```python
from build123d import *

# Parameters (mm, degrees)
F2_T     = -30.48
F3_DEPTH = 50.8
F4_R     = 12.7


with BuildPart() as f1:
    # F0 (on Front) → F1 (revolve)
    with BuildSketch(Plane.XZ):
        Polygon((-152.4, 0), (0, 0), (0, 152.4), (-208.28, 152.4), align=None)
    revolve(axis=Axis((0, 0, 76.2), (0, 0, -1)))

    # F2
    f2_openings = [f1.faces().sort_by_distance(p)[0] for p in [
        (0, 0, 152.4),
    ]]
    offset(amount=F2_T, openings=f2_openings)

    # F3 (add): a face of the model
    f3_faces = [f1.faces().sort_by_distance(p)[0] for p in [
        (202.3889519846, 0, 152.4),
    ]]
    extrude(f3_faces, amount=F3_DEPTH)

    # F4
    f4_edges = [f1.edges().sort_by_distance(p)[0] for p in [
        (208.28, 0, 203.2),
        (175.81566, 0, 203.2),
        (175.81566, 0, 152.4),
        (208.28, 0, 152.4),
        (152.4, 0, 0),
    ]]
    fillet(f4_edges, radius=F4_R)


solid = f1.part
```
Check sheet for the modelled part. Datum: model origin and axes. Units: mm. A direction names the side the tool comes from. Round coordinates to 2 decimals unless told otherwise and drop trailing zeros. Order: outer loops, then holes, each group sorted by start corner. A loop starts at its lowest first (then second) coordinate and runs counter-clockwise, first axis right, second up. Notation, with made-up numbers: (50, 8) -> (54, 8) arc R33 cw to (54, 43) -> close; hole circle Ø7 at (78, 75). An arc over 180 degrees is marked (long way). Use CSV: the item, a comma, the result in double quotes.
(1) Cross-section at B-B (z = 113). Record the boundary of the cut face in (x, y), and give its area (3 significant figures).
Worked out:
outline,"circle Ø387.67 at (0, 0); hole circle Ø322.74 at (0, 0)"
area,"36,200 mm²"
(2) Cross-section at A-A (z = 169). Record the boundary of the cut face in (x, y).
Worked out:
outline,"circle Ø416.56 at (0, 0); hole circle Ø351.63 at (0, 0)"
(3) Depth check by flat-ended pin: pin 1 (1 mm diameter, centred on y = 159.5, z = 151, fed in from +X); pin 2 (1.5 mm diameter, centred on y = -148.5, z = 94.5, fed in from +X); pin 3 (12 mm diameter, centred on y = 43, z = 142.5, fed in from +X). Enter the tip coordinate at first touch or a pass-through.
Worked out:
pin 1,"x = 133.74"
pin 2,"x = 114.81"
pin 3,"x = 202.65"
(4) Tool access check on faces 1 (the face through (-102, 160, 203.2)), 2 (the face through (2, 2, 30.48)). Record the directions out of +Z, -Z, +X, -X, +Y, -Y that give a thin tool (end or side, any length) a straight path to the whole face; none if there is none.
Worked out:
face 1,"+Z, +X, -X, +Y, -Y"
face 2,"+Z"
(5) Draft check along X on faces 3 (the face through (2, 2, 0)), 4 (the face through (-167.7, 52.8, 172.3)), 5 (the face through (27.11, 206.51, 172.33)). Enter one of: pulls with the +X half, pulls with the -X half, needs draft (parallel to the pull), parting line crosses it, or undercut.
Worked out:
face 3,"needs draft"
face 4,"undercut"
face 5,"parting line crosses it"
(6) Material ranges on line 1 along Y through (x, z) = (0, 172); line 2 along Z through (x, y) = (57.5, 47.5), recorded low to high. Write a range as from..to.
Worked out:
line 1,"-208.28..-175.82, 175.82..208.28"
line 2,"0..30.48"
